Geometry: see drawing. Coordinates: mm, zero at the bounding-box minimum. A direction names the side the tool comes from. Coordinates: 2 decimals unless noted, no trailing zeros. Loops run counter-clockwise (first coordinate to the right, second up) from the corner with the lowest first, then second, coordinate; pieces in that order, holes last. Notation, with made-up numbers: (-20.5, -37) -> (-12.5, -37) arc R15 cw to (-12.5, -9) -> close; hole circle Ø11 at (41.25, 84). An arc over 180 degrees is marked (long way). Answer as a JSON object with one key per item and string values.
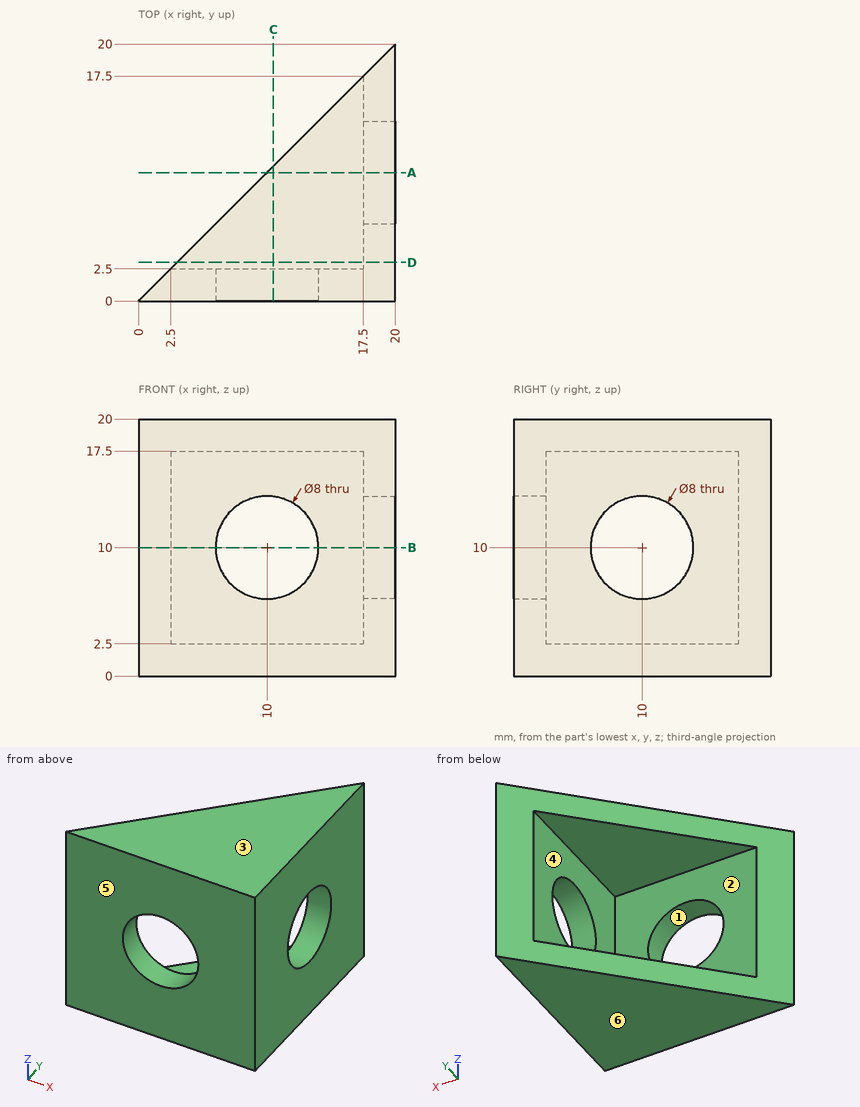
1. Section query D-D (y = 3). Return loops of the section in (x, z), plus the area to 4 significant figures.
Reply:
{"outline": "(3, 0) -> (20, 0) -> (20, 20) -> (3, 20) -> (3, 17.5) -> (17.5, 17.5) -> (17.5, 2.5) -> (3, 2.5) -> close", "area": "122.5 mm2"}
2. Access query for the marked faces 1 and 2. Directions: +Z, -Z, +X, -X, +Y, -Y. A direction counts if a zero-diameter tool reaches every point of the face in a straight line with its end or side. Return the directions, or none.
Reply:
{"face 1": "+Y, -Y", "face 2": "-X, +Y"}
3. Section query C-C (x = 10.5). Return loops of the section in (y, z).
Reply:
{"outline": "(0, 0) -> (10.5, 0) -> (10.5, 2.5) -> (2.5, 2.5) -> (2.5, 6.03) -> (0, 6.03) -> close; (0, 13.97) -> (2.5, 13.97) -> (2.5, 17.5) -> (10.5, 17.5) -> (10.5, 20) -> (0, 20) -> close"}
4. Section query A-A (y = 10). Return loops of the section in (x, z), plus the area to 3 significant figures.
Reply:
{"outline": "(10, 0) -> (20, 0) -> (20, 6) -> (17.5, 6) -> (17.5, 2.5) -> (10, 2.5) -> close; (10, 17.5) -> (17.5, 17.5) -> (17.5, 14) -> (20, 14) -> (20, 20) -> (10, 20) -> close", "area": "67.5 mm2"}
5. Pin query (flat end, axial travel): P1, Ø4, axis at x = 12, y = 16.5, coming from the +Z side; P2, Ø1.5, axis at x = 2.5, z = 16.5, coming from the +Y side; P3, Ø3, axis at x = 13.5, z = 2.5, coming from the +Y side; P4, Ø1, axis at y = 12.5, z = 2.5, coming from the -X side. Return the tip coordinate at first contact, or that it passes through.
Reply:
{"P1": "passes through", "P2": "stops at y = 2.5", "P3": "stops at y = 15", "P4": "stops at x = 12"}
6. Line query: line 1 along Z through (x, y) = (16.25, 7.5); line 2 along X through (y, z) = (8, 3); line 3 along X through (y, z) = (0.9, 10). Output: solid intervals per line, ascending.
Reply:
{"line 1": "z = 0 to 2.5, 17.5 to 20", "line 2": "x = 17.5 to 20", "line 3": "x = 0.9 to 6, 14 to 20"}
7. Mould query, pull axis Z, two halves, no side actions, for the marked faces 3, 4, 5 and 6. Classes: pulls with the +Z half, pulls with the -Z half, needs draft (parallel to the pull), parting line crosses it, or undercut.
Reply:
{"face 3": "pulls with the +Z half", "face 4": "undercut", "face 5": "needs draft", "face 6": "pulls with the -Z half"}
8. Section query B-B (z = 10). Return loops of the section in (x, y), plus the area to 3 significant figures.
Reply:
{"outline": "(0, 0) -> (6, 0) -> (6, 2.5) -> (2.5, 2.5) -> close; (14, 0) -> (20, 0) -> (20, 6) -> (17.5, 6) -> (17.5, 2.5) -> (14, 2.5) -> close; (17.5, 14) -> (20, 14) -> (20, 20) -> (17.5, 17.5) -> close", "area": "47.5 mm2"}
